Could you check a few things on this drawing? It's one solid part, dimensions in mm from its lowest x, y, z. Round coordinates to 2 decimals unless told otherwise and drop trailing zeros. Order: outer loops, then holes, each group sorted by start corner. A loop starts at its lowest first (then second) coordinate and runs counter-clockwise, first axis right, second up. Notation, with made-up numbers: (41.25, 35.25) -> (93.25, 35.25) arc R16 ccw to (93.25, 55.25) -> close; hole circle Ø11 at (-2, 55.5). An arc over 180 degrees is marked (long way). Use a Markdown table: item, result. Add a question column.
(1) I want a section at C-C, the plane y = 5.75. Please give me the cut outline in (x, z) (1 decimal).
(2) I want a section at A-A, the plane y = 2. Give the number of separate pieces and of enclosed holes in the cut face, then the cut area to 3 significant figures.
(3) I'm going to push flat-ended pins straight in: P1, Ø3, axis at x = 7.05, y = 3.18, coming from the -Z side; P2, Ø3, axis at y = 3, z = 8.5, coming from the -X side. Where does each tip first touch, or does it pass through?
(4) If I drill on probe 1 along X at (y, z) = (3, 3.75) (1 decimal); probe 2 along X at (y, z) = (2, 6); probe 3 along Z at (x, y) = (51.5, 4) (1 decimal), over which ranges is the centre line in solid material (lowest first)?
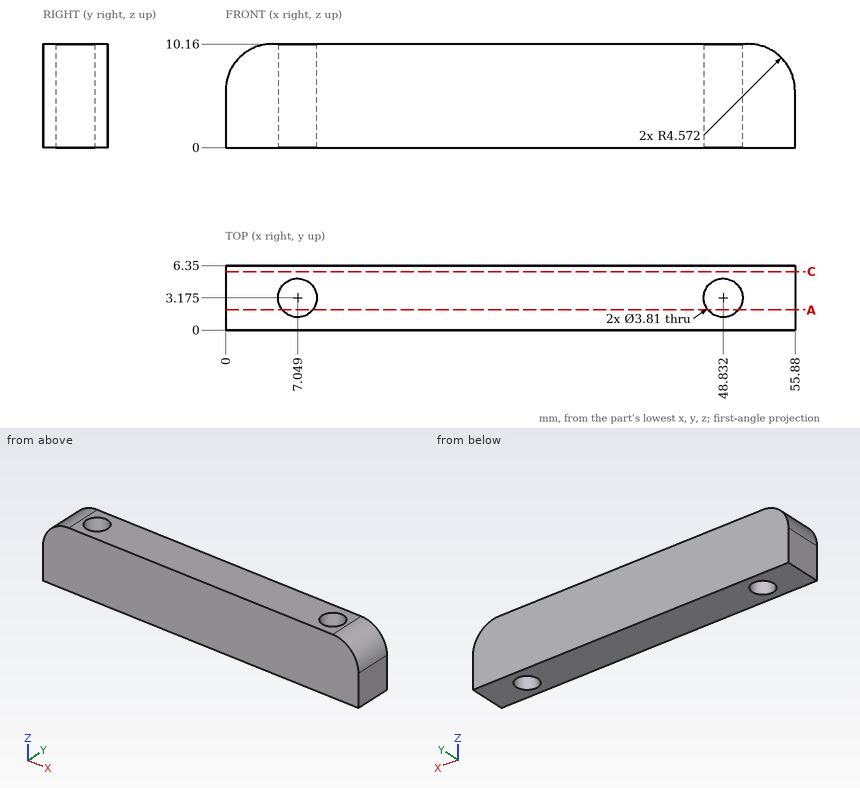
Taken from the geometry:
| question | item | result |
|---|---|---|
| 1 | outline | (0, 0) -> (55.9, 0) -> (55.9, 5.6) arc R4.6 ccw to (51.3, 10.2) -> (4.6, 10.2) arc R4.6 ccw to (0, 5.6) -> close |
| 2 | separate pieces | 3 |
| 2 | enclosed holes | 0 |
| 2 | area | 498 mm2 |
| 3 | P1 | passes through |
| 3 | P2 | stops at x = 0.22 |
| 4 | probe 1 | x = 0 to 5.2, 8.9 to 46.9, 50.7 to 55.9 |
| 4 | probe 2 | x = 0.02 to 5.55, 8.55 to 47.33, 50.33 to 55.86 |
| 4 | probe 3 | z = 0 to 10.2 |
